Read the model definition and answer for the solid it produces. Units are mm, in the model's axes. A direction names the side the tool comes from. Coordinates: 2 decimals unless noted, no trailing zeros. Loops run counter-clockwise (first coordinate to the right, second up) from the corner with the lowest first, then second, coordinate; pieces in that order, holes last. Notation, with made-up numbers: M 52,-39.75 L 96,-39.75 A26 ccw 96,-21.75 Z; hole C 50,57 d8. An arc over 180 degrees is marked long. Put each result on its own line as item: value.
from build123d import *

# Parameters (mm, degrees)
F1_DEPTH    = 500
F2_T1_DEPTH = 359.4621544115
F3_T1_DEPTH = 359.4621544115


# Not quite as in the source:
# - a fillet or chamfer that OpenCascade refuses, or shapes differently, is made with other operations: its cross-section is extruded or revolved along the edge and cut away or added


with BuildPart() as f1:
    # F0 (on Front) → F1 (new body, symmetric)
    with BuildSketch(Plane.XZ):
        Polygon((50, -7.6415093219), (50, 7.6415093219), (-50, 7.6415093219), (-50, -7.6415093219), (-10.5660382013, -7.6415093219), (-1.1320764027, -7.6415093219), (0, -7.6415093219), (9.4339617987, -7.6415093219), align=None)
        Polygon((9.4339617987, -57.6415093219), (9.4339617987, -7.6415093219), (0, -7.6415093219), (-1.1320764027, -7.6415093219), (-10.5660382013, -7.6415093219), (-10.5660382013, -57.6415093219), align=None)
    extrude(amount=F1_DEPTH, both=True)

    # F2: chamfer of 66 on 1 edges, made by hand

    # F2_s2 → F2_t1 (cut)
    with BuildSketch(Plane.YZ.offset(-180.2971154071)):
        Polygon((434, -57.6415093219), (500, 8.3584906781), (500, -57.6415093219), align=None)
    extrude(amount=F2_T1_DEPTH, mode=Mode.SUBTRACT)

    # F3: chamfer of 66 on 1 edges, made by hand

    # F3_s2 → F3_t1 (cut)
    with BuildSketch(Plane.YZ.offset(-180.2971154071)):
        Polygon((-500, 8.3584906781), (-434, -57.6415093219), (-500, -57.6415093219), align=None)
    extrude(amount=F3_T1_DEPTH, mode=Mode.SUBTRACT)


solid = f1.part
1) Given pin 1 Ø15 at (y, z) = (191.5, -21.5) entering from -X; pin 2 Ø6 at (x, y) = (-35.5, 385) entering from -Z; pin 3 Ø2 at (y, z) = (198.5, -46) entering from +X, each flat-ended and moving along its own axis, determine where each tip first touches the part or whether it passes through.
Answer list:
pin 1: stops at x = -10.57
pin 2: stops at z = -7.64
pin 3: stops at x = 9.43
2) Straight lines are drawn through the part: line 1 (X direction, y = -122, z = -11); line 2 (Z direction, x = 18, y = 337); line 3 (Y direction, x = 42, z = -7). For each, find the intervals that lie inside material, in ascending order. Write a range as [from, to].
Answer list:
line 1: x = [-10.57, 9.43]
line 2: z = [-7.64, 7.64]
line 3: y = [-484.64, 484.64]
3) Which of the six approach directions +Z, -Z, +X, -X, +Y, -Y give full straight-line access (tool end or side, diameter ignored) to faces 1 (the flat face through (9.434, -7, -33)), 2 (the flat face through (50, -7, 0)), 3 (the flat face through (-31, -7, -7.642))?
Answer list:
face 1: -Z, +X, +Y, -Y
face 2: +Z, -Z, +X, +Y, -Y
face 3: -Z, -X, +Y, -Y
4) Find section A-A, the plane y = -60. Write down the section's boundary in (x, z), plus the area to 3 significant figures.
Answer list:
outline: M -50,-7.64 L -10.57,-7.64 L -10.57,-57.64 L 9.43,-57.64 L 9.43,-7.64 L 50,-7.64 L 50,7.64 L -50,7.64 Z
area: 2,530 mm^2
5) Find section C-C, the plane z = -32. Write down the section's boundary in (x, y), plus the area to 3 significant figures.
Answer list:
outline: M -10.57,-459.64 L 9.43,-459.64 L 9.43,459.64 L -10.57,459.64 Z
area: 18,400 mm^2
6) Find section B-B, the plane x = 35.5. Write down the section's boundary in (y, z).
Answer list:
outline: M -499.28,7.64 L -484,-7.64 L 484,-7.64 L 499.28,7.64 Z
